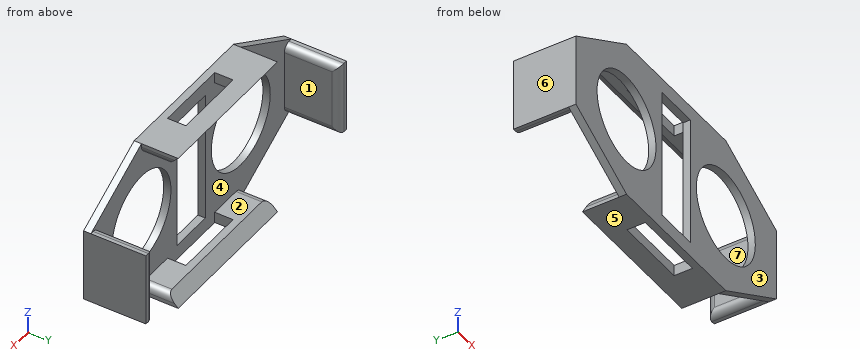
from build123d import *

# Parameters (mm, degrees)
SKETCH1_W           = 85
SKETCH1_H           = 44
BOSS_EXTRUDE1_DEPTH = 2
SKETCH2_W           = 3
SKETCH2_H           = 20
BOSS_EXTRUDE2_DEPTH = 15
SKETCH3_W           = 42.103313086
SKETCH3_H           = 3
BOSS_EXTRUDE3_DEPTH = 10
SKETCH4_W           = 20
SKETCH4_H           = 5
CUT_EXTRUDE1_DEPTH  = 99.208960895
CHAMFER1_SIZE       = 3
FILLET1_R           = 2
SKETCH6_OUTSIDE_W   = 106.442
SKETCH6_OUTSIDE_H   = 65.442
SKETCH6_OUTSIDE_R   = 12.5
SKETCH6_OUTSIDE_W_2 = 12
SKETCH6_OUTSIDE_H_2 = 36
CUT_EXTRUDE3_DEPTH  = 2


with BuildPart() as part:
    # Sketch1 → Boss-Extrude1 (new body)
    with BuildSketch(Plane(origin=(0, 5, 0), x_dir=(1, 0, 0), z_dir=(0, 1, 0))):
        with Locations((42.5, 22)):
            Rectangle(SKETCH1_W, SKETCH1_H)
    extrude(amount=BOSS_EXTRUDE1_DEPTH)

    # Sketch2 → Boss-Extrude2 (add)
    with BuildSketch(Plane(origin=(0, 7, 0), x_dir=(1, 0, 0), z_dir=(0, 1, 0))):
        with Locations((1.5, 22)):
            Rectangle(SKETCH2_W, SKETCH2_H)
        with Locations((83.5, 22)):
            Rectangle(SKETCH2_W, SKETCH2_H)
    extrude(amount=BOSS_EXTRUDE2_DEPTH)

    # Sketch3 → Boss-Extrude3 (add)
    with BuildSketch(Plane(origin=(0, 7, 0), x_dir=(1, 0, 0), z_dir=(0, 1, 0))):
        with Locations((42.5, 42.5)):
            Rectangle(SKETCH3_W, SKETCH3_H)
        with Locations((42.5, 1.5)):
            Rectangle(SKETCH3_W, SKETCH3_H)
    extrude(amount=BOSS_EXTRUDE3_DEPTH)

    # Sketch4 → Cut-Extrude1 (cut, through all)
    with BuildSketch(Plane.XY):
        with Locations((42.5, 9.5)):
            Rectangle(SKETCH4_W, SKETCH4_H)
    extrude(amount=-CUT_EXTRUDE1_DEPTH, mode=Mode.SUBTRACT)

    # Chamfer1
    chamfer1_edges = [part.edges().sort_by_distance(p)[0] for p in [
        (42.5, 17, -3),
        (42.5, 17, -41),
    ]]
    chamfer(chamfer1_edges, length=CHAMFER1_SIZE - 0.0001)  # a hair under: the kernel refuses the full size

    # Fillet1
    fillet1_edges = [part.edges().sort_by_distance(p)[0] for p in [
        (3, 14.5, -12),
        (3, 14.5, -32),
        (3, 22, -22),
        (82, 14.5, -32),
        (82, 14.5, -12),
        (82, 22, -22),
        (0, 6, -44),
        (85, 6, -44),
        (85, 6, 0),
        (0, 6, 0),
        (21.448343457, 10.50005, -3),
        (63.551656543, 10.50005, -3),
        (63.551656543, 10.50005, -41),
        (21.448343457, 10.50005, -41),
    ]]
    fillet(fillet1_edges, radius=FILLET1_R)

    # Sketch6 outside → Cut-Extrude3 (cut)
    # profile 1 of 4: a face of its own
    with BuildSketch(Plane(origin=(0, 5, 0), x_dir=(1, 0, 0), z_dir=(0, 1, 0))):
        with Locations((42.5, 22)):
            Rectangle(SKETCH6_OUTSIDE_W, SKETCH6_OUTSIDE_H)
        Polygon((0, 32), (21.448343457, 44), (63.551656543, 44), (85, 32), (85, 12), (63.551656543, 0), (21.448343457, 0), (0, 12), align=None, mode=Mode.SUBTRACT)
    # profile 2 of 4: a face of its own
    with BuildSketch(Plane(origin=(0, 5, 0), x_dir=(1, 0, 0), z_dir=(0, 1, 0))):
        with Locations(Location((21.448343457, 22, 0), (0, 0, 90))):
            Circle(SKETCH6_OUTSIDE_R)
    # profile 3 of 4: a face of its own
    with BuildSketch(Plane(origin=(0, 5, 0), x_dir=(1, 0, 0), z_dir=(0, 1, 0))):
        with Locations(Location((63.551656543, 22, 0), (0, 0, 90))):
            Circle(SKETCH6_OUTSIDE_R)
    # profile 4 of 4: a face of its own
    with BuildSketch(Plane(origin=(0, 5, 0), x_dir=(1, 0, 0), z_dir=(0, 1, 0))):
        with Locations((42.5, 22)):
            Rectangle(SKETCH6_OUTSIDE_W_2, SKETCH6_OUTSIDE_H_2)
    extrude(amount=CUT_EXTRUDE3_DEPTH, mode=Mode.SUBTRACT)


solid = part.part
Work out the finished part from the listing and answer in its coordinate system (mm). Face numbers are marked on the shaded views. A direction names the side the tool comes from. Coordinates: 2 decimals unless noted, no trailing zeros. Write each loop counter-clockwise with the first axis right and the second up, starting at its lowest first coordinate (ties: lowest second). Pieces come first, ordered by that corner, then holes. Notation, with made-up numbers: M 82,8.25 L 109,8.25 A30 cw 109,31.25 Z; hole C 87.25,31 d9. An arc over 180 degrees is marked long. Answer as CSV lines item,"result". Start each with the question number.
Item 1: Determine the mould class of the marked faces 4, 5, 6 and 7 for opening direction X: released by +X, released by -X, zero draft, split by the parting line, or undercut.
Item 2: Flat-ended cylindrical pins translate along their axes: P1, Ø1.5, axis at y = 9, z = -1, coming from the +X side; P2, Ø0.9, axis at y = 9, z = -2, coming from the -X side; P3, Ø1.1, axis at y = 13, z = -0.5, coming from the -X side. Find the tip coordinate at first contact, or state that the pin passes through.
Item 3: Section C-C on x = 35.5 is taken. Give the number of separate pieces and of enclosed holes in the cut face, and give its area (3 significant figures).
Item 4: Section A-A on z = -22 is taken. Write down the section's boundary in (x, y), and give its area (3 significant figures).
Item 5: Consider L1, parallel to Z at x = 29, y = 13.75; L2, parallel to X at y = 11.25, z = -23.5; L3, parallel to Y at x = 69.5, z = -7. Determine where each line is inside the solid, lowest interval first.
Item 6: Section B-B on y = 18 is taken. Write down the section's boundary in (x, z), and give its area (3 significant figures).
Item 7: A tool of negligible diameter and unlimited length cuts with its end or side. For the marked faces 1, 2 and 3, from which of +Z, -Z, +X, -X, +Y, -Y can it reach the whole face along a straight path? Write none if from no direction.
Checks:
1,face 4,"undercut"
1,face 5,"zero draft"
1,face 6,"released by -X"
1,face 7,"undercut"
2,P1,"stops at x = 63.55"
2,P2,"stops at x = 21.53"
2,P3,"stops at x = 21.45"
3,separate pieces,"3"
3,enclosed holes,"0"
3,area,"109 mm²"
4,outline,"M 0,5 L 8.95,5 L 8.95,7 L 3,7 L 3,20 A2 ccw 1,22 L 0,22 Z; M 33.95,5 L 36.5,5 L 36.5,7 L 33.95,7 Z; M 48.5,5 L 51.05,5 L 51.05,7 L 48.5,7 Z; M 76.05,5 L 85,5 L 85,22 L 84,22 A2 ccw 82,20 L 82,7 L 76.05,7 Z"
4,area,"134 mm²"
5,L1,"z = -44 to -41, -3 to 0"
5,L2,"x = 0 to 3, 82 to 85"
5,L3,"y = 5 to 7"
6,outline,"M 0,-32 L 1,-32 A2 ccw 3,-30 L 3,-14 A2 ccw 1,-12 L 0,-12 Z; M 82,-30 A2 ccw 84,-32 L 85,-32 L 85,-12 L 84,-12 A2 ccw 82,-14 Z"
6,area,"117 mm²"
7,face 1,"+Z, -Z, +Y"
7,face 2,"+X, -X, +Y"
7,face 3,"+Z, -Z, +X, -X, -Y"
